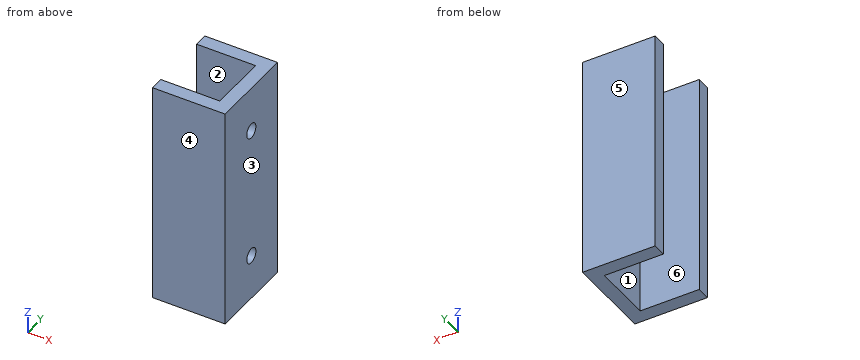
from build123d import *

# Parameters (mm, degrees)
SKETCH_1_W          = 19
SKETCH_1_H          = 19
SKETCH_1_W_2        = 13
SKETCH_1_H_2        = 13
EXTRUDE_1_DEPTH     = 49.33
SKETCH_2_R          = 1.65
CUT_EXTRUDE_1_DEPTH = 30
SKETCH_3_W          = 116.915177823
SKETCH_3_H          = 46.219516436
CUT_EXTRUDE_2_DEPTH = 3


with BuildPart() as part:
    # 草图1 → Extrude 1 (new body)
    with BuildSketch(Plane.XY):
        with Locations((6.5, 6.5)):
            Rectangle(SKETCH_1_W, SKETCH_1_H)
        with Locations((6.5, 6.5)):
            Rectangle(SKETCH_1_W_2, SKETCH_1_H_2, mode=Mode.SUBTRACT)
    extrude(amount=EXTRUDE_1_DEPTH)

    # 草图2 → 切除-拉伸1 (cut)
    with BuildSketch(Plane.ZY.offset(3)):
        with Locations((10, 6.5)):
            Circle(SKETCH_2_R)
        with Locations((39.33, 6.5)):
            Circle(SKETCH_2_R)
    extrude(amount=-CUT_EXTRUDE_1_DEPTH, mode=Mode.SUBTRACT)

    # 草图3 → 切除-拉伸2 (cut)
    with BuildSketch(Plane.ZY.offset(3)):
        with Locations((53.162237228, 0.202739406)):
            Rectangle(SKETCH_3_W, SKETCH_3_H)
    extrude(amount=-CUT_EXTRUDE_2_DEPTH, mode=Mode.SUBTRACT)


solid = part.part
Check sheet for the modelled part. Datum: model origin and axes. Units: mm. Face numbers are marked on the shaded views. A direction names the side the tool comes from. Round coordinates to 2 decimals unless told otherwise and drop trailing zeros. Order: outer loops, then holes, each group sorted by start corner. A loop starts at its lowest first (then second) coordinate and runs counter-clockwise, first axis right, second up.
Q1. Set-up check for the marked faces 5 and 6: record each of +Z, -Z, +X, -X, +Y, -Y from which the full face is reachable in a straight line by a thin tool's end or side.
Filled sheet:
face 5: +Z, -Z, +X, -X, +Y
face 6: +Z, -Z, -X
Q2. Draft check along Y on the marked faces 1, 2, 3 and 4. Enter one of: pulls with the +Y half, pulls with the -Y half, needs draft (parallel to the pull), parting line crosses it, or undercut.
Filled sheet:
face 1: undercut
face 2: undercut
face 3: needs draft
face 4: pulls with the -Y half
Q3. Cross-section at B-B, the plane x = 11.75. Enter the section's corners in (y, z).
Filled sheet:
outline: (-3, 0) - (0, 0) - (0, 49.33) - (-3, 49.33) - close; (13, 0) - (16, 0) - (16, 49.33) - (13, 49.33) - close
Q4. Cross-section at C-C, the plane y = 6.5. Enter the section's corners in (x, z).
Filled sheet:
outline: (13, 0) - (16, 0) - (16, 8.35) - (13, 8.35) - close; (13, 11.65) - (16, 11.65) - (16, 37.68) - (13, 37.68) - close; (13, 40.98) - (16, 40.98) - (16, 49.33) - (13, 49.33) - close
Q5. Cross-section at A-A, the plane z = 10. Enter the section's corners in (x, y), plus the area to 3 significant figures.
Filled sheet:
outline: (0, -3) - (16, -3) - (16, 4.85) - (13, 4.85) - (13, 0) - (0, 0) - close; (0, 13) - (13, 13) - (13, 8.15) - (16, 8.15) - (16, 16) - (0, 16) - close
area: 125 mm2
Q6. Cross-section at D-D, the plane x = 13.75. Enter the section's corners in (y, z).
Filled sheet:
outline: (-3, 0) - (16, 0) - (16, 49.33) - (-3, 49.33) - close; hole circle Ø3.3 at (6.5, 10); hole circle Ø3.3 at (6.5, 39.33)
Q7. Scan lines: L1, parallel to Y at x = 9.5, z = 46.5; L2, parallel to Y at x = 14.75, z = 39.33; L3, parallel to X at y = 6.5, z = 28.5. Record each from-to range of solid material in increasing order.
Filled sheet:
L1: y = -3 to 0, 13 to 16
L2: y = -3 to 4.85, 8.15 to 16
L3: x = 13 to 16
Q8. Depth check by flat-ended pin: P1, Ø4, axis at y = 8.5, z = 44, coming from the -X side; P2, Ø4, axis at x = 4.5, y = 10, coming from the -Z side. Enter the tip coordinate at first touch or a pass-through.
Filled sheet:
P1: stops at x = 13
P2: passes through
